Source: CAD feature listing. Evaluate the final solid. Frame: model axes, mm. Give positions to 0.01 mm unless a question says otherwise; leave off trailing zeros. Use CSV: the item, a comma, the result in double quotes.
```python
from build123d import *

# Parameters (mm, degrees)
FILLET1_R       = 0.2032
HEX_2_DEPTH     = 0.9652
THDSCHPAT_COUNT = 20
THDSCHPAT_PITCH = 0.453517


with BuildPart() as part:
    # BodySke → Base-Revolve (revolve)
    with BuildSketch(Plane.XY):
        Polygon((0, 0), (0, 1.5494), (0.2286, 1.778), (2.1844, 1.778), (2.1844, 1.0922), (11.44016, 1.0922), (11.7094, 0.82296), (11.7094, 0), align=None)
    revolve(axis=Axis((-31.75, 0, 0), (1, 0, 0)))

    # Fillet1
    fillet1_edges = [part.edges().sort_by_distance(p)[0] for p in [
        (2.1844, -1.0922, 0),
    ]]
    fillet(fillet1_edges, radius=FILLET1_R)

    # Sketch2 → Hex-PreBroach (revolve, cut)
    with BuildSketch(Plane.XY):
        Polygon((0, 0.9906), (0.9652, 0.9906), (1.537123177, 0), (0, 0), align=None)
    revolve(axis=Axis((0, 0, 0), (1, 0, 0)), mode=Mode.SUBTRACT)

    # Sketch3 → Hex 2 (cut)
    with BuildSketch(Plane(origin=(0, 0, 0), x_dir=(0, 0.5, 0.866025404), z_dir=(-1, 0, 0))):
        Polygon((0.571923177, 0.9906), (-0.571923177, 0.9906), (-1.143846353, 0), (-0.571923177, -0.9906), (0.571923177, -0.9906), (1.143846353, 0), align=None)
    extrude(amount=-HEX_2_DEPTH, mode=Mode.SUBTRACT)

    # ThdSchSke → ThreadSchematic (revolve, cut)
    with BuildSketch(Plane.XY):
        Polygon((2.63906, -0.82296), (2.450536122, -1.0922), (2.450536122, -1.36525), (2.827583878, -1.36525), (2.827583878, -1.0922), align=None)
    threadschematic = revolve(axis=Axis((-3.175, 0, 0), (1, 0, 0)), mode=Mode.SUBTRACT)

    # ThdSchPat: ThreadSchematic ×20
    with Locations(*[(i * THDSCHPAT_PITCH, 0, 0) for i in range(1, THDSCHPAT_COUNT)]):
        add(threadschematic, mode=Mode.SUBTRACT)


solid = part.part
```
Item 1: Material intervals for line 1 (Y direction, x = 0.5, z = 0.15); line 2 (X direction, y = 1.25, z = -0.5); line 3 (Z direction, x = 5, y = -0.3), sorted ascending. Write a range as from..to.
Filled in:
line 1,"y = -1.77..-1.06, 1.06..1.77"
line 2,"x = 0..2.18"
line 3,"z = -0.91..0.91"
Item 2: Mould query, pull axis Z, two halves, no side actions, for faces 1 (the conical face through (1.446, -0.126, -0.096)), 2 (the flat face through (11.709, 0, 0)). Classes: released by +Z, released by -Z, zero draft, split by the parting line, or undercut.
Filled in:
face 1,"undercut"
face 2,"zero draft"
Item 3: First-contact query: pin 1 (1.5 mm diameter, centred on x = 5.5, z = -0.5, fed in from +Y); pin 2 (1.5 mm diameter, centred on x = 10, y = -0.5, fed in from +Z); pin 3 (1.5 mm diameter, centred on x = 6, z = -1, fed in from -Y). Flat tips, straight axial feed; report the tip coordinate or a pass-through.
Filled in:
pin 1,"stops at y = 1.09"
pin 2,"stops at z = 1.09"
pin 3,"stops at y = -1.06"
